The listing builds one solid part. Answer for the finished solid, in the listing's coordinates (mm). Face numbers are marked on the shaded views. A direction names the side the tool comes from. Give positions to 0.01 mm unless a question says otherwise; leave off trailing zeros. Order: outer loops, then holes, each group sorted by start corner. A loop starts at its lowest first (then second) coordinate and runs counter-clockwise, first axis right, second up.
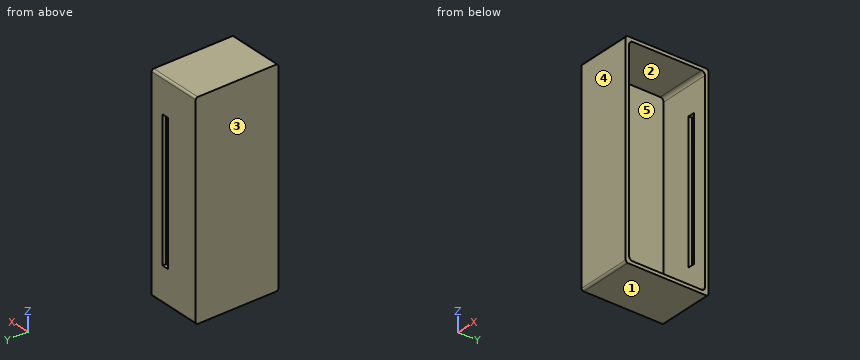
```python
from build123d import *

# Parameters (mm, degrees)
SKETCH_1_W          = 300
SKETCH_1_H          = 120
EXTRUDE_1_DEPTH     = 80
FILLET_1_R          = 3
SHELL_1_T           = -5
FILLET_2_R          = 5
SKETCH_3_W          = 10
SKETCH_3_H          = 200
CUT_EXTRUDE_1_DEPTH = 5


with BuildPart() as part:
    # 草图1 → 凸台-拉伸1 (new body)
    with BuildSketch(Plane(origin=(0, 0, 0), x_dir=(0, 0, -1), z_dir=(1, 0, 0))):
        with Locations((3.008457619, 67.850176247)):
            Rectangle(SKETCH_1_W, SKETCH_1_H)
    extrude(amount=EXTRUDE_1_DEPTH)

    # 圆角1
    fillet_1_edges = [part.edges().sort_by_distance(p)[0] for p in [
        (40, 127.850176247, 146.991542381),
        (40, 127.850176247, -153.008457619),
        (40, 7.850176247, -153.008457619),
        (40, 7.850176247, 146.991542381),
    ]]
    fillet(fillet_1_edges, radius=FILLET_1_R)

    # 抽壳1
    shell_1_openings = [part.faces().sort_by_distance(p)[0] for p in [
        (80, 67.850176247, -3.008457619),
    ]]
    offset(amount=SHELL_1_T, openings=shell_1_openings, kind=Kind.INTERSECTION)

    # 圆角2
    fillet_2_edges = [part.edges().sort_by_distance(p)[0] for p in [
        (42.5, 12.850176247, 141.991542381),
        (42.5, 12.850176247, -148.008457619),
        (42.5, 122.850176247, -148.008457619),
        (42.5, 122.850176247, 141.991542381),
    ]]
    fillet(fillet_2_edges, radius=FILLET_2_R)

    # 草图3 → 切除-拉伸1 (cut)
    with BuildSketch(Plane(origin=(0, 127.850176247, 0), x_dir=(1, 0, 0), z_dir=(0, 1, 0))):
        with Locations((55, 3.008457619)):
            Rectangle(SKETCH_3_W, SKETCH_3_H)
    extrude(amount=-CUT_EXTRUDE_1_DEPTH, mode=Mode.SUBTRACT)


solid = part.part
```
1) Find section D-D (y = 96). Write down the section's boundary in (x, z), then the cut area to 3 significant figures.
Geometry says:
outline: (0, -153.01) - (80, -153.01) - (80, -148.01) - (5, -148.01) - (5, 141.99) - (80, 141.99) - (80, 146.99) - (0, 146.99) - close
area: 2,250 mm2
2) Straight lines are drawn through the part: probe 1 along Y at (x, z) = (10.5, -34.5); probe 2 along Z at (x, y) = (40.5, 44.5); probe 3 along X at (y, z) = (19.5, -130.5). For each, find the intervals that lie inside material, in ascending order.
Geometry says:
probe 1: y = 7.85 to 12.85, 122.85 to 127.85
probe 2: z = -153.01 to -148.01, 141.99 to 146.99
probe 3: x = 0 to 5
3) Given P1, Ø1.5, axis at x = 56.5, y = 126, coming from the -Z side; P2, Ø2, axis at y = 37, z = 105.5, coming from the +X side, each flat-ended and moving along its own axis, determine where each tip first touches the part or whether it passes through.
Geometry says:
P1: stops at z = -152.98
P2: stops at x = 5
4) For a pull along Z with two mould halves and no side action, classify the marked faces 1, 2 and 3 as +Z half, -Z half, draft (parallel to the pull), parting line (faces both ways), or undercut.
Geometry says:
face 1: -Z half
face 2: undercut
face 3: draft
5) Find section B-B (z = 38). Write down the section's boundary in (x, y), then the cut area to 3 significant figures.
Geometry says:
outline: (0, 7.85) - (80, 7.85) - (80, 12.85) - (5, 12.85) - (5, 122.85) - (50, 122.85) - (50, 127.85) - (0, 127.85) - close; (60, 122.85) - (80, 122.85) - (80, 127.85) - (60, 127.85) - close
area: 1,300 mm2
6) Find section A-A (x = 74). Write down the section's boundary in (y, z).
Geometry says:
outline: (7.85, -150.01) arc R3 ccw to (10.85, -153.01) - (124.85, -153.01) arc R3 ccw to (127.85, -150.01) - (127.85, 143.99) arc R3 ccw to (124.85, 146.99) - (10.85, 146.99) arc R3 ccw to (7.85, 143.99) - close; hole (12.85, -143.01) arc R5 ccw to (17.85, -148.01) - (117.85, -148.01) arc R5 ccw to (122.85, -143.01) - (122.85, 136.99) arc R5 ccw to (117.85, 141.99) - (17.85, 141.99) arc R5 ccw to (12.85, 136.99) - close
7) A tool of negligible diameter and unlimited length cuts with its end or side. For the marked faces 4 and 5, from which of +Z, -Z, +X, -X, +Y, -Y can it reach the whole face along a straight path? Write none if from no direction.
Geometry says:
face 4: +Z, -Z, +X, -X, -Y
face 5: +X
8) Find section C-C (z = 126.5). Write down the section's boundary in (x, y), then the cut area to 3 significant figures.
Geometry says:
outline: (0, 7.85) - (80, 7.85) - (80, 12.85) - (5, 12.85) - (5, 122.85) - (80, 122.85) - (80, 127.85) - (0, 127.85) - close
area: 1,350 mm2
